Job drawing, mm, ordinate dimensions from the low corner. One solid piece. A direction names the side the tool comes from. Round coordinates to 2 decimals unless told otherwise and drop trailing zeros. Write each loop counter-clockwise with the first axis right and the second up, starting at its lowest first coordinate (ties: lowest second). Pieces come first, ordered by that corner, then holes. Notation, with made-up numbers: (48, -31) -> (60, -31) arc R18 ccw to (60, -9) -> close; hole circle Ø7 at (21, 47). An arc over 180 degrees is marked (long way). Use CSV: the item, a comma, the result in double quotes. Start each with the question number.
(1) Saw through at C-C (z = 11). Give the cut face in (x, y), plus the area to 3 significant figures.
(2) Probe line 1 (Y direction, x = 55, z = 3.75); line 2 (Y direction, x = 55, z = 15); line 3 (X direction, y = 62.5, z = 18). List the from-to ranges inside material, lowest first. Write a range as [from, to].
(3) Drop flat-ended pins along their axis: pin 1 (10 mm diameter, centred on x = 28, z = 16.5, fed in from +Y); pin 2 (12 mm diameter, centred on x = 30.5, z = 4.5, fed in from +Y); pin 3 (10 mm diameter, centred on x = 97, z = 22, fed in from +Y). Give the stop position or say it passes through.
(4) Saw through at A-A (y = 55). Give the cut face in (x, z).
(5) Saw through at D-D (z = 17). Give the cut face in (x, y), plus the area to 3 significant figures.
(6) Which spindle directions (+Z, -Z, +X, -X, +Y, -Y) get a long thin tool onto all of the face, cutting with end or side? Do the marked faces 1 and 2. Say none if no direction does.
(7) Two-plate mould, pull along Y, no slides. Class the marked faces 3, 4 and 5: released by +Y, released by -Y, zero draft, split by the parting line, or undercut.
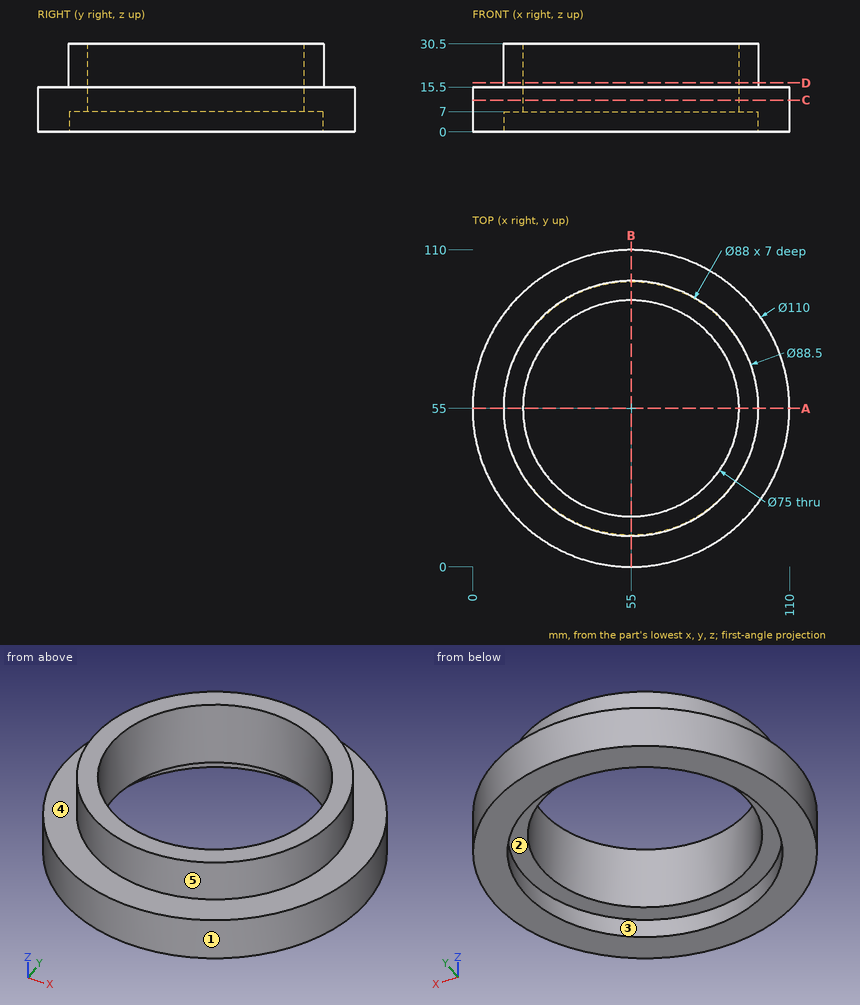
Answers:
1,outline,"circle Ø110 at (55, 55); hole circle Ø75 at (55, 55)"
1,area,"5,090 mm²"
2,line 1,"y = [0, 11], [99, 110]"
2,line 2,"y = [0, 17.5], [92.5, 110]"
2,line 3,"x = [11.39, 18.26], [91.74, 98.61]"
3,pin 1,"stops at y = 105.36"
3,pin 2,"stops at y = 106.8"
3,pin 3,"stops at y = 79.27"
4,outline,"(0, 0) -> (11, 0) -> (11, 7) -> (17.5, 7) -> (17.5, 30.5) -> (10.75, 30.5) -> (10.75, 15.5) -> (0, 15.5) -> close; (92.5, 7) -> (99, 7) -> (99, 0) -> (110, 0) -> (110, 15.5) -> (99.25, 15.5) -> (99.25, 30.5) -> (92.5, 30.5) -> close"
5,outline,"circle Ø88.5 at (55, 55); hole circle Ø75 at (55, 55)"
5,area,"1,730 mm²"
6,face 1,"+Z, -Z"
6,face 2,"-Z"
7,face 3,"undercut"
7,face 4,"zero draft"
7,face 5,"split by the parting line"
